from build123d import *


with BuildPart() as part:
    # Sketch1 → Revolve1 (revolve)
    with BuildSketch(Plane(origin=(0, 0, 0), x_dir=(0, 0, -1), z_dir=(1, 0, 0)), mode=Mode.PRIVATE) as revolve1_sk:
        with BuildLine():
            Line((-3.37, 8.375), (-1.515544457, 8.375))
            ThreePointArc((-1.515544457, 8.375), (0, 9.25), (1.515544457, 8.375))
            Line((1.515544457, 8.375), (3.37, 8.375))
            Line((3.37, 8.375), (3.5, 8.505))
            Line((3.5, 8.505), (3.5, 10.74))
            ThreePointArc((3.5, 10.74), (3.423847763, 10.923847763), (3.24, 11))
            Line((3.24, 11), (-3.24, 11))
            ThreePointArc((-3.24, 11), (-3.423847763, 10.923847763), (-3.5, 10.74))
            Line((-3.5, 10.74), (-3.5, 8.505))
            Line((-3.5, 8.505), (-3.37, 8.375))
        make_face()
    revolve(revolve1_sk.sketch.rotate(Axis((0, 0, 3.5), (0, 0, -1)), 90), axis=Axis((0, 0, 3.5), (0, 0, -1)))


solid = part.part
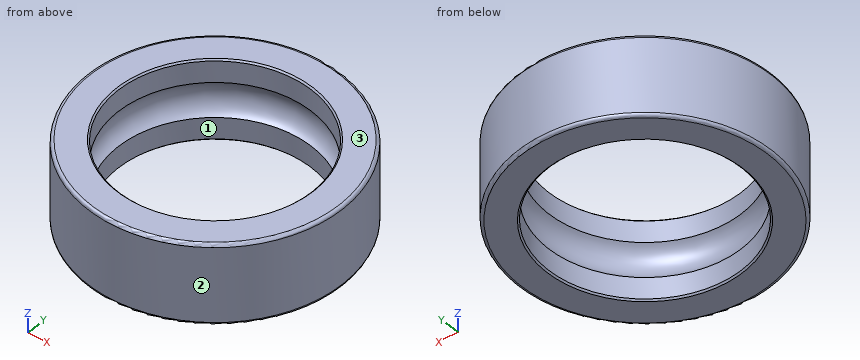
Input: part model. Units: mm. Frame: model coordinates. Face numbers are marked on the shaded views. Coordinates: 2 decimals unless noted, no trailing zeros. Loops run counter-clockwise (first coordinate to the right, second up) from the corner with the lowest first, then second, coordinate; pieces in that order, holes last. Notation, with made-up numbers: (79, 85) - (107, 85) arc R8 cw to (107, 97) - close; hole circle Ø1 at (26.5, 42). An arc over 180 degrees is marked (long way). Answer in a Markdown table with one row per item. Add a question column.
Item 1: Section query C-C on z = -2.25. Return the cut outline in (x, y) (3 decimals), then the cut area to 3 significant figures.
Item 2: Contact query for flat-ended pins moving along their axis: P1, Ø1.5, axis at x = 5, z = -0.5, coming from the +Y side; P2, Ø2, axis at x = 2.5, y = 5.5, coming from the -Z side; P3, Ø12, axis at x = -6.5, y = 3, coming from the +Z side; P4, Ø2, axis at x = 5, z = 1, coming from the -Y side. Output: stop coordinate, or through.
Item 3: Section query A-A on x = 0. Return the cut outline in (y, z) (3 decimals), then the cut area to 3 significant figures.
Item 4: Line query: line 1 along Y through (x, z) = (0, 1.95) (3 decimals); line 2 along X through (y, z) = (-6.5, 2.25); line 3 along Y through (x, z) = (-3.5, 3). Output: solid intervals per line, ascending. Write a range as [from, to].
Item 5: Mould query, pull axis Y, two halves, no side actions, for the marked faces 1, 2 and 3. Classes: released by +Y, released by -Y, zero draft, split by the parting line, or undercut.
Recorded:
| question | item | result |
|---|---|---|
| 1 | outline | circle Ø22 at (0, 0); hole circle Ø16.75 at (0, 0) |
| 1 | area | 160 mm^2 |
| 2 | P1 | y = 10.15 |
| 2 | P2 | through |
| 2 | P3 | z = 3.5 |
| 2 | P4 | y = -10.25 |
| 3 | outline | (-11, -3.24) arc R0.26 ccw to (-10.74, -3.5) - (-8.505, -3.5) - (-8.375, -3.37) - (-8.375, -1.516) arc R1.75 cw to (-8.375, 1.516) - (-8.375, 3.37) - (-8.505, 3.5) - (-10.74, 3.5) arc R0.26 ccw to (-11, 3.24) - close; (8.375, -3.37) - (8.505, -3.5) - (10.74, -3.5) arc R0.26 ccw to (11, -3.24) - (11, 3.24) arc R0.26 ccw to (10.74, 3.5) - (8.505, 3.5) - (8.375, 3.37) - (8.375, 1.516) arc R1.75 cw to (8.375, -1.516) - close |
| 3 | area | 32.9 mm^2 |
| 4 | line 1 | [-11, -8.375], [8.375, 11] |
| 4 | line 2 | [-8.87, -5.28], [5.28, 8.87] |
| 4 | line 3 | [-10.43, -7.61], [7.61, 10.43] |
| 5 | face 1 | undercut |
| 5 | face 2 | split by the parting line |
| 5 | face 3 | zero draft |
